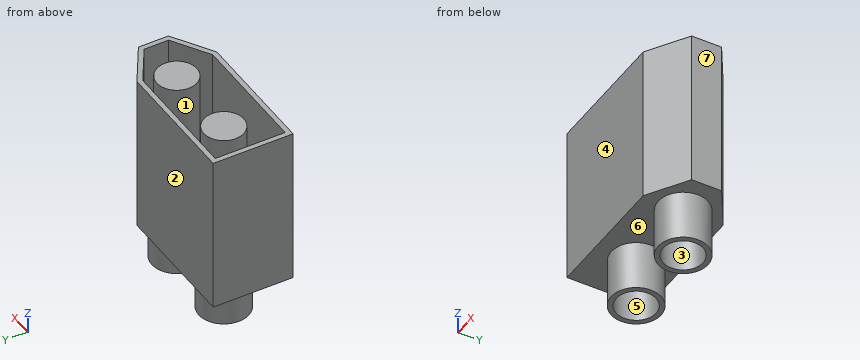
from build123d import *

# Parameters (mm, degrees)
F1_DEPTH = 6
F3_DEPTH = 10
F4_R     = 2.5
F5_DEPTH = 5
F6_R     = 2
F7_DEPTH = 5
F8_R     = 2
F9_DEPTH = 9


with BuildPart() as f1:
    # F0 (on Top) → F1 (new body)
    with BuildSketch(Plane.XY):
        Polygon((-13, 0.832660675), (-13, -7.167339325), (0, -7.167339325), (4, -4.667339325), (4, -1.667339325), (0, 0.832660675), align=None)
    extrude(amount=F1_DEPTH)

    # F2 (on face) → F3 (join)
    with BuildSketch(Plane.XY.offset(6)):
        Polygon((0, 0.832660675), (-13, 0.832660675), (-13, -7.167339325), (0, -7.167339325), (4, -4.667339325), (4, -1.667339325), align=None)
        Polygon((-12.5, 0.332660675), (-0.1433981132, 0.332660675), (3.5, -1.9444631457), (3.5, -4.3902155042), (-0.1433981132, -6.667339325), (-12.5, -6.667339325), align=None, mode=Mode.SUBTRACT)
    extrude(amount=F3_DEPTH)

    # F4 (on face) → F5 (join)
    with BuildSketch(Plane(origin=(0, 0, 0), x_dir=(1, 0, 0), z_dir=(0, 0, -1))):
        with Locations((0, 3.167339325)):
            Circle(F4_R)
        with Locations((-8, 3.167339325)):
            Circle(F4_R)
    extrude(amount=F5_DEPTH)

    # F6 (on face) → F7 (cut)
    with BuildSketch(Plane(origin=(0, 0, -5), x_dir=(1, 0, 0), z_dir=(0, 0, -1))):
        with Locations((-8, 3.167339325)):
            Circle(F6_R)
        with Locations((0, 3.167339325)):
            Circle(F6_R)
    extrude(amount=-F7_DEPTH, mode=Mode.SUBTRACT)

    # F8 (on face) → F9 (join)
    with BuildSketch(Plane.XY.offset(6)):
        with Locations((-8, -3.167339325)):
            Circle(F8_R)
        with Locations((0, -3.167339325)):
            Circle(F8_R)
    extrude(amount=F9_DEPTH)


solid = f1.part
Source: CAD feature listing. Evaluate the final solid. Frame: model axes, mm. Face numbers are marked on the shaded views. A direction names the side the tool comes from. Give positions to 0.01 mm unless a question says otherwise; leave off trailing zeros. Write each loop counter-clockwise with the first axis right and the second up, starting at its lowest first coordinate (ties: lowest second). Pieces come first, ordered by that corner, then holes. Notation, with made-up numbers: M -22,82 L 8,82 A31 ccw 8,106 Z; hole C 63,-18.75 d8. An arc over 180 degrees is marked long. Return JSON: item names as keys, results as strings. Group by question number.
1) First-contact query: pin 1 Ø2 at (x, y) = (0.5, -2.5) entering from -Z; pin 2 Ø4.5 at (x, y) = (-8, -3.17) entering from +Z; pin 3 Ø1.5 at (y, z) = (-4.5, -2.5) entering from -X. Flat tips, straight axial feed; report the tip coordinate or a pass-through.
2) Cut plane C-C, the plane z = 2. Output: boundary loops of the cut face in (x, y).
3) Ray query, L1, parallel to Y at x = 0, z = -1; L2, parallel to X at y = -3.5, z = 7; L3, parallel to X at y = -2.5, z = 6.5. Return the intervals inside material, ascending.
4) Draft query along X for the marked faces 4, 5, 6 and 7. Return one class per face: released by +X, released by -X, zero draft, split by the parting line, or undercut.
5) Set-up query: the marked faces 1, 2 and 3. Return all of +Z, -Z, +X, -X, +Y, -Y with unobstructed straight access to the full face (end or side cutting, diameter ignored); none if empty.
6) Cut plane B-B, the plane x = -8. Output: boundary loops of the cut face in (y, z), then the cut area to 3 significant figures.
7) Cut plane D-D, the plane z = -2.75. Output: boundary loops of the cut face in (x, y), then the cut area to 3 significant figures.
8) Cut plane A-A, the plane z = 12.5. Output: boundary loops of the cut face in (x, y), then the cut area to 3 significant figures.
Data:
{
 "1": {"pin 1": "stops at z = 0", "pin 2": "stops at z = 15", "pin 3": "stops at x = -10.43"},
 "2": {"outline": "M -13,-7.17 L 0,-7.17 L 4,-4.67 L 4,-1.67 L 0,0.83 L -13,0.83 Z"},
 "3": {"L1": "y = -5.67 to -5.17, -1.17 to -0.67", "L2": "x = -13 to -12.5, -9.97 to -6.03, -1.97 to 1.97, 3.5 to 4", "L3": "x = -13 to -12.5, -9.89 to -6.11, -1.89 to 1.89, 3.5 to 4"},
 "4": {"face 4": "zero draft", "face 5": "undercut", "face 6": "undercut", "face 7": "released by +X"},
 "5": {"face 1": "+Z", "face 2": "+Z, -Z, +X, -X, +Y", "face 3": "-Z"},
 "6": {"outline": "M -7.17,0 L -5.67,0 L -5.67,-5 L -5.17,-5 L -5.17,0 L -1.17,0 L -1.17,-5 L -0.67,-5 L -0.67,0 L 0.83,0 L 0.83,16 L 0.33,16 L 0.33,6 L -1.17,6 L -1.17,15 L -5.17,15 L -5.17,6 L -6.67,6 L -6.67,16 L -7.17,16 Z", "area": "99.0 mm²"},
 "7": {"outline": "C -8,-3.17 d5; C 0,-3.17 d5; hole C -8,-3.17 d4; hole C 0,-3.17 d4", "area": "14.1 mm²"},
 "8": {"outline": "M -13,-7.17 L 0,-7.17 L 4,-4.67 L 4,-1.67 L 0,0.83 L -13,0.83 Z; C -8,-3.17 d4; C 0,-3.17 d4; hole M -12.5,-6.67 L -0.14,-6.67 L 3.5,-4.39 L 3.5,-1.94 L -0.14,0.33 L -12.5,0.33 Z", "area": "47.4 mm²"}
}
